from build123d import *

# Parameters (mm, degrees)
F0_W          = 19.2
F0_H          = 19.2
F1_DEPTH      = 1.8
F3_DEPTH      = 3
F5_DEPTH      = 3
F7_DEPTH      = 2
F7_DEPTH_BACK = 2
F9_DEPTH      = 2
F9_DEPTH_BACK = 2


with BuildPart() as f1:
    # F0 (on Top) → F1 (new body)
    with BuildSketch(Plane.XY):
        Rectangle(F0_W, F0_H)
    extrude(amount=F1_DEPTH)

    # F2 (on face) → F3 (cut)
    with BuildSketch(Plane.XZ.offset(9.6)):
        Polygon((-2.01, 1.15), (-1.36, 1.8), (-9.6, 1.8), (-9.6, 1.15), align=None)
        Polygon((0.57, 1.8), (-0.57, 1.8), (-0.37, 1.6), (0.37, 1.6), align=None)
        Polygon((9.6, 1.8), (1.36, 1.8), (2.01, 1.15), (9.6, 1.15), align=None)
    extrude(amount=-F3_DEPTH, mode=Mode.SUBTRACT)

    # F4 (on face) → F5 (cut)
    with BuildSketch(Plane(origin=(0, 9.6, 0), x_dir=(-1, 0, 0), z_dir=(0, 1, 0))):
        Polygon((-9.6, 1.8), (-9.6, 1.15), (-2.03, 1.15), (-1.38, 1.8), align=None)
        Polygon((0.57, 1.8), (-0.57, 1.8), (-0.37, 1.6), (0.37, 1.6), align=None)
        Polygon((2.03, 1.15), (9.6, 1.15), (9.6, 1.8), (1.38, 1.8), align=None)
    extrude(amount=-F5_DEPTH, mode=Mode.SUBTRACT)

    # F6 (on Front) → F7 (join, two sides)
    with BuildSketch(Plane.XZ) as f7_sk:
        Polygon((-5.75, 4.4), (-5.75, 0), (-5, 0), (-5, 3.7), (-4.25, 3.4), (-4.25, 4.4), align=None)
        Polygon((4.25, 3.4), (5, 3.7), (5, 0), (5.75, 0), (5.75, 4.4), (4.25, 4.4), align=None)
    extrude(amount=F7_DEPTH)
    extrude(f7_sk.sketch, amount=-F7_DEPTH_BACK)

    # F8 (on Right) → F9 (join, two sides)
    with BuildSketch(Plane.YZ) as f9_sk:
        Polygon((-5.75, 4.4), (-5.75, 0), (-5, 0), (-5, 3.7), (-4.25, 3.4), (-4.25, 4.4), align=None)
        Polygon((4.25, 4.4), (4.25, 3.4), (5, 3.7), (5, 0), (5.75, 0), (5.75, 4.4), align=None)
    extrude(amount=F9_DEPTH)
    extrude(f9_sk.sketch, amount=-F9_DEPTH_BACK)


solid = f1.part
Design review of the part built by this model. Coordinates are the model's own, in mm. A direction names the side the tool comes from. Round coordinates to 2 decimals unless told otherwise and drop trailing zeros. Write each loop counter-clockwise with the first axis right and the second up, starting at its lowest first coordinate (ties: lowest second). Pieces come first, ordered by that corner, then holes. Notation, with made-up numbers: M 26,-39 L 53,-39 A14 ccw 53,-18 Z; hole C 65,-10.5 d10. An arc over 180 degrees is marked long. One line per item, written item: value. Start each with the question number.
1. For faces 1 (the face through (5.2, -2, 3.4)), 2 (the face through (6, -8, 1.15)), 3 (the face through (-5.75, 0, 3)), 4 (the face through (5, 0, 3)), list the 3-axis set-ups (+Z, -Z, +X, -X, +Y, -Y) from which the entire face can be reached by the end or side of a thin tool; tool diameter is ignored.
2. To check wall thickness, follow probe 1 along Y at (x, z) = (1.25, 2.25); probe 2 along Z at (x, y) = (4.75, 4); probe 3 along Z at (x, y) = (-0.25, -7.25). State the ranges of each line that lie inside material, in increasing order. Write a range as from..to.
3. Take a section at C-C on y = -8.25. State the section outline as (x, z) points.
4. Take a section at D-D on y = 0.25. State the section outline as (x, z) points.
5. Draft analysis for pull direction Y (two halves, no side actions). For faces 5 (the face through (0, 5.75, 3)), 6 (the face through (-4.25, 0, 4)), 7 (the face through (0, 0, 1.8)), state which applies: pulls with the +Y half, pulls with the -Y half, needs draft (parallel to the pull), parting line crosses it, or undercut.
6. Take a section at A-A on z = 3. State the section outline as (x, y) points.
7. Clearance check with flat-ended pins moving along their axes: P1, Ø1, axis at x = 0, z = 2.5, coming from the -Y side; P2, Ø0.8, axis at x = 0, y = 8, coming from the +Z side; P3, Ø2.5, axis at x = 5, y = 7.5, coming from the +Z side. State where each tip first meets the part, or that it passes through.
8. Take a section at B-B on x = -4. State the section outline as (y, z) points, then the cut area to 3 significant figures.
Computed:
1. face 1: +Z, +X, -X, -Y
1. face 2: +Z, +X, -Y
1. face 3: +Z, -X, +Y, -Y
1. face 4: +Y, -Y
2. probe 1: y = -5.75..-5, 5..5.75
2. probe 2: z = 0..1.8
2. probe 3: z = 0..1.6
3. outline: M -9.6,0 L 9.6,0 L 9.6,1.15 L 2.01,1.15 L 1.36,1.8 L 0.57,1.8 L 0.37,1.6 L -0.37,1.6 L -0.57,1.8 L -1.36,1.8 L -2.01,1.15 L -9.6,1.15 Z
4. outline: M -9.6,0 L 9.6,0 L 9.6,1.8 L 5.75,1.8 L 5.75,4.4 L 4.25,4.4 L 4.25,3.4 L 5,3.7 L 5,1.8 L -5,1.8 L -5,3.7 L -4.25,3.4 L -4.25,4.4 L -5.75,4.4 L -5.75,1.8 L -9.6,1.8 Z
5. face 5: pulls with the +Y half
5. face 6: needs draft
5. face 7: undercut
6. outline: M -5.75,-2 L -5,-2 L -5,2 L -5.75,2 Z; M -2,-5.75 L 2,-5.75 L 2,-5 L -2,-5 Z; M -2,5 L 2,5 L 2,5.75 L -2,5.75 Z; M 5,-2 L 5.75,-2 L 5.75,2 L 5,2 Z
7. P1: stops at y = -5.75
7. P2: stops at z = 1.63
7. P3: stops at z = 1.8
8. outline: M -9.6,0 L 9.6,0 L 9.6,1.15 L 6.6,1.15 L 6.6,1.8 L -6.6,1.8 L -6.6,1.15 L -9.6,1.15 Z
8. area: 30.7 mm²
